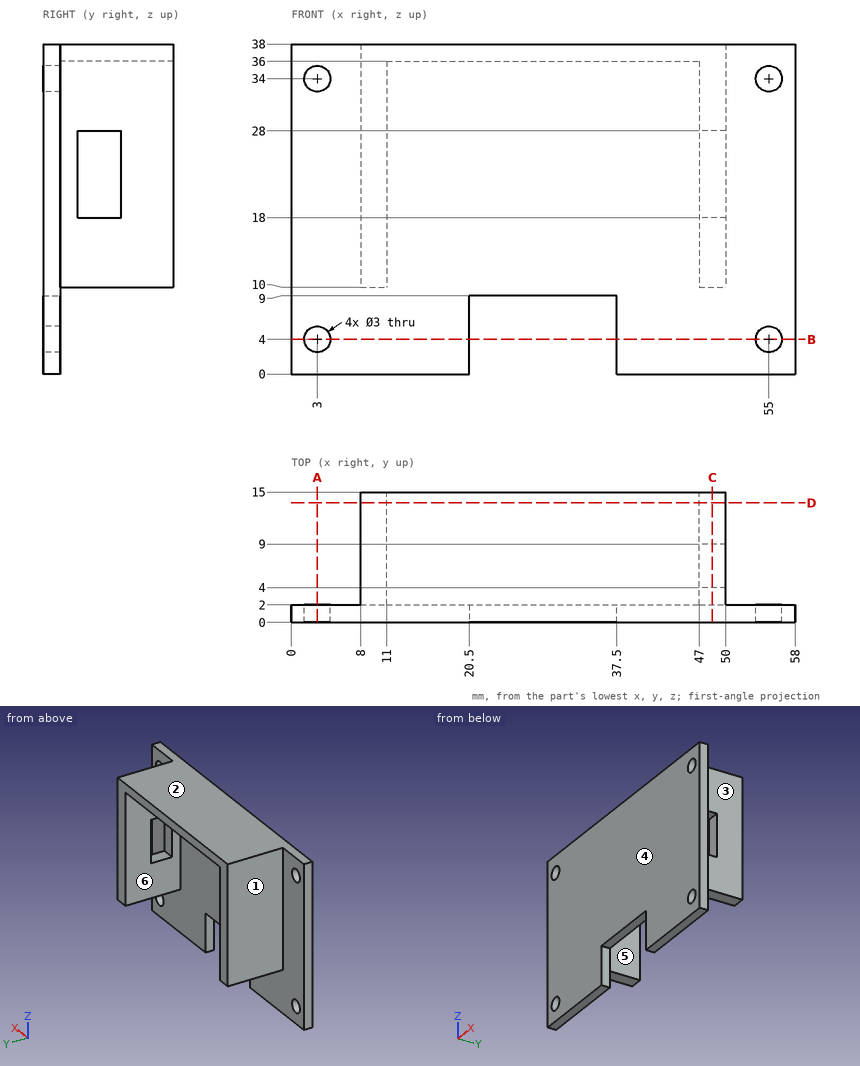
Job drawing, mm, ordinate dimensions from the low corner. One solid piece. A direction names the side the tool comes from. Give positions to 0.01 mm unless a question says otherwise; leave off trailing zeros. Loops run counter-clockwise (first coordinate to the right, second up) from the corner with the lowest first, then second, coordinate; pieces in that order, holes last. Notation, with made-up numbers: M 0,-8 L 25,-8 A9 cw 25,9 Z; hole C 35,53 d1. An arc over 180 degrees is marked long. Put each result on its own line as item: value. Start each with the question number.
1) Saw through at C-C (x = 48.5). List the corners of the cut face in (y, z), then the cut area to 3 significant figures.
2) Saw through at D-D (y = 13.75). List the corners of the cut face in (x, z), then the cut area to 3 significant figures.
3) Probe probe 1 along X at (y, z) = (0.8, 4); probe 2 along X at (y, z) = (1.1, 34); probe 3 along X at (y, z) = (4.75, 34). List the from-to ranges inside material, lowest first.
4) Pull direction X, two halves, no side cores. Call the marked faces 3, 4, 5 and 6: +X half, -X half, draft (parallel to the pull), parting line (faces both ways), or undercut.
5) Flat gauge pins, fed straight in: pin 1 (1.5 mm diameter, centred on x = 49, y = 6, fed in from -Z); pin 2 (8 mm diameter, centred on y = 8.5, z = 13.5, fed in from -X); pin 3 (4 mm diameter, centred on y = 8.5, z = 25.5, fed in from +X); pin 4 (4 mm diameter, centred on x = 26, z = 25.5, fed in from -Y). Where does each tip first touch, or does it go through?
6) Saw through at A-A (x = 3). List the corners of the cut face in (y, z), then the cut area to 3 significant figures.
7) Saw through at B-B (z = 4). List the corners of the cut face in (x, y), then the cut area to 3 significant figures.
8) 3-axis set-ups, long thin cutter, end or side, ignore diameter. For the marked faces 1 and 2: which of +Z, -Z, +X, -X, +Y, -Y reach the whole face in a straight line?
Numbers:
1. outline: M 0,0 L 2,0 L 2,10 L 15,10 L 15,38 L 0,38 Z; hole M 4,18 L 9,18 L 9,28 L 4,28 Z
1. area: 390 mm^2
2. outline: M 8,10 L 11,10 L 11,36 L 47,36 L 47,10 L 50,10 L 50,38 L 8,38 Z
2. area: 240 mm^2
3. probe 1: 0 to 1.5, 4.5 to 20.5, 37.5 to 53.5, 56.5 to 58
3. probe 2: 0 to 1.5, 4.5 to 53.5, 56.5 to 58
3. probe 3: 8 to 11, 47 to 50
4. face 3: +X half
4. face 4: draft
4. face 5: undercut
4. face 6: undercut
5. pin 1: z = 10
5. pin 2: x = 8
5. pin 3: x = 50
5. pin 4: y = 0
6. outline: M 0,0 L 2,0 L 2,2.5 L 0,2.5 Z; M 0,5.5 L 2,5.5 L 2,32.5 L 0,32.5 Z; M 0,35.5 L 2,35.5 L 2,38 L 0,38 Z
6. area: 64.0 mm^2
7. outline: M 0,0 L 1.5,0 L 1.5,2 L 0,2 Z; M 4.5,0 L 20.5,0 L 20.5,2 L 4.5,2 Z; M 37.5,0 L 53.5,0 L 53.5,2 L 37.5,2 Z; M 56.5,0 L 58,0 L 58,2 L 56.5,2 Z
7. area: 70.0 mm^2
8. face 1: +Z, -Z, -X, +Y
8. face 2: +Z, +X, -X, +Y, -Y
